Read the model definition and answer for the solid it produces. Units are mm, in the model's axes. A direction names the side the tool comes from. Give positions to 0.01 mm unless a question says otherwise; leave off trailing zeros. Write each loop counter-clockwise with the first axis right and the second up, starting at its lowest first coordinate (ties: lowest second). Pieces come first, ordered by that corner, then holes. Notation, with made-up numbers: M -24.5,46 L -20.5,46 A11 cw -20.5,52 Z; hole C 24.5,64.25 d11. An arc over 180 degrees is marked long. Put each result on its own line as item: value.
from build123d import *

# Parameters (mm, degrees)
BOSS_EXTRUDE1_DEPTH  = 11.25
CUT_EXTRUDE1_DEPTH   = 10
M3_CLEARANCE_HOLE1_D = 3.4
SKETCH7_W            = 5.75
SKETCH7_H            = 4
CUT_EXTRUDE2_DEPTH   = 10


with BuildPart() as part:
    # Sketch1 → Boss-Extrude1 (new body)
    with BuildSketch(Plane(origin=(0, 0, 0), x_dir=(0, 0, -1), z_dir=(1, 0, 0))):
        with BuildLine():
            Line((-24, 0.5), (-24, -0.5))
            ThreePointArc((-24, -0.5), (-22.828427125, -3.328427125), (-20, -4.5))
            Line((-20, -4.5), (20, -4.5))
            ThreePointArc((20, -4.5), (22.828427125, -3.328427125), (24, -0.5))
            Line((24, -0.5), (24, 0.5))
            ThreePointArc((24, 0.5), (22.828427125, 3.328427125), (20, 4.5))
            Line((20, 4.5), (-20, 4.5))
            ThreePointArc((-20, 4.5), (-22.828427125, 3.328427125), (-24, 0.5))
        make_face()
    extrude(amount=BOSS_EXTRUDE1_DEPTH)

    # Sketch2 → Cut-Extrude1 (cut, through all)
    with BuildSketch(Plane(origin=(0, -4.5, 0), x_dir=(-1, 0, 0), z_dir=(0, -1, 0))):
        with BuildLine():
            Line((-2, -3.25), (0, -3.25))
            Line((0, -3.25), (0, 3.25))
            Line((0, 3.25), (-2, 3.25))
            ThreePointArc((-2, 3.25), (-5.25, 0), (-2, -3.25))
        make_face()
    extrude(amount=-CUT_EXTRUDE1_DEPTH, mode=Mode.SUBTRACT)

    # M3 Clearance Hole1 (through all)
    with Locations(Plane(origin=(11.25, 0, 0), x_dir=(0, 0, -1), z_dir=(1, 0, 0))):
        with Locations((-20, 0), (20, 0)):
            Hole(M3_CLEARANCE_HOLE1_D / 2)

    # Sketch7 → Cut-Extrude2 (cut, through all)
    with BuildSketch(Plane(origin=(0, -4.5, 0), x_dir=(-1, 0, 0), z_dir=(0, -1, 0))):
        with Locations((-8.375, -22)):
            Rectangle(SKETCH7_W, SKETCH7_H)
        with BuildLine():
            Line((-11.25, -20), (-5.5, -20))
            Line((-5.5, -20), (-5.5, -16))
            ThreePointArc((-5.5, -16), (-9.768861754, -8.500919068), (-11.25, 0))
            Line((-11.25, 0), (-11.25, -20))
        make_face()
        with BuildLine():
            Line((-11.25, 20), (-11.25, 0))
            ThreePointArc((-11.25, 0), (-9.768861754, 8.500919068), (-5.5, 16))
            Line((-5.5, 16), (-5.5, 20))
            Line((-5.5, 20), (-11.25, 20))
        make_face()
        with Locations((-8.375, 22)):
            Rectangle(SKETCH7_W, SKETCH7_H)
    extrude(amount=-CUT_EXTRUDE2_DEPTH, mode=Mode.SUBTRACT)


solid = part.part
(1) Section B-B on z = -15.5 is taken. Determine the outline of the cut face in (x, y), and give its area (3 significant figures).
Result:
outline: M 0,-4.5 L 5.9,-4.5 L 5.9,4.5 L 0,4.5 Z
area: 53.1 mm²
(2) Section C-C on x = 8 is taken. Determine the outline of the cut face in (y, z).
Result:
outline: M -4.5,-12.36 L 4.5,-12.36 L 4.5,12.36 L -4.5,12.36 Z
(3) For a pull along Y with two mould halves and no side action, classify faces 1 (the face through (2.712, 3.359, 22.797)), 2 (the face through (2.71, -0.65, 21.57)), 3 (the face through (1, 0, 3.25)), 4 (the face through (6, -4.5, 0)) as +Y half, -Y half, draft (parallel to the pull), parting line (faces both ways), or undercut.
Result:
face 1: +Y half
face 2: undercut
face 3: draft
face 4: -Y half
(4) Which of the six approach directions +Z, -Z, +X, -X, +Y, -Y give full straight-line access (tool end or side, diameter ignored) to faces 5 (the face through (5.5, 0, 18)), 6 (the face through (5.5, 0, -18)), 7 (the face through (1, 0, -3.25))?
Result:
face 5: +Z, +X, +Y, -Y
face 6: -Z, +X, +Y, -Y
face 7: -X, +Y, -Y
(5) Straight lines are drawn through the part: line 1 along Y through (x, z) = (2.7, -20); line 2 along X through (y, z) = (1.5, 21); line 3 along Z through (x, y) = (0.5, -1.5). For each, find the intervals that lie inside material, in ascending order. Write a range as from..to.
Result:
line 1: y = -4.5..-1.7, 1.7..4.5
line 2: x = 0..5.5
line 3: z = -23.87..-20.8, -19.2..-3.25, 3.25..19.2, 20.8..23.87
(6) Given pin 1 Ø2 at (y, z) = (0, -20) entering from -X; pin 2 Ø1 at (y, z) = (0.5, 2.5) entering from -X; pin 3 Ø4 at (y, z) = (-3, 3.5) entering from +X; pin 4 Ø1 at (x, y) = (0.5, 2) entering from +Z, each flat-ended and moving along its own axis, determine where each tip first touches the part or whether it passes through.
Result:
pin 1: passes through
pin 2: stops at x = 3.25
pin 3: stops at x = 11.21
pin 4: stops at z = 23.87
(7) Section A-A on y = 2.5 is taken. Determine the outline of the cut face in (x, z).
Result:
outline: M 0,-23.46 L 5.5,-23.46 L 5.5,-16 A25.14 ccw 5.5,16 L 5.5,23.46 L 0,23.46 L 0,3.25 L 2,3.25 A3.25 cw 2,-3.25 L 0,-3.25 Z
